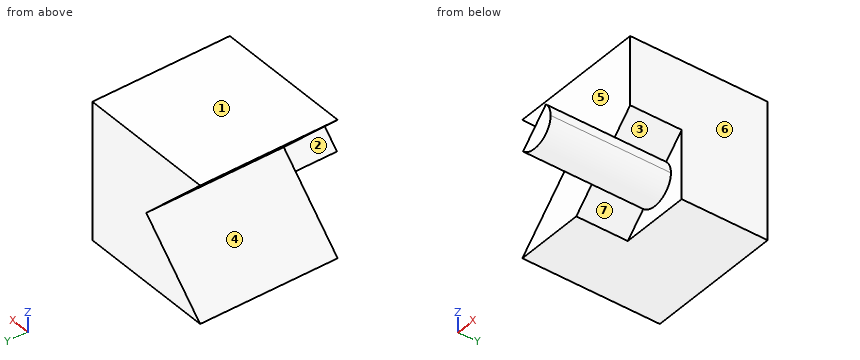
from build123d import *

# Parameters (mm, degrees)
F1_DEPTH = 40
F2_DEPTH = 25
F3_DEPTH = 60


with BuildPart() as f1:
    # F0 (on Front) → F1 (new body)
    with BuildSketch(Plane.XZ):
        with BuildLine():
            Line((20, 20), (0, 0))
            Line((0, 0), (20, 0))
            Line((20, 0), (25.7573593129, 5.7573593129))
            ThreePointArc((25.7573593129, 5.7573593129), (25.7573593129, 14.2426406871), (34.2426406871, 14.2426406871))
            Line((34.2426406871, 14.2426406871), (40, 20))
            Line((40, 20), (40, 40))
            Line((40, 40), (0, 40))
            Line((0, 40), (20, 20))
        make_face()
        with BuildLine():
            ThreePointArc((34.2426406871, 14.2426406871), (25.7573593129, 14.2426406871), (25.7573593129, 5.7573593129))
            Line((25.7573593129, 5.7573593129), (34.2426406871, 14.2426406871))
        make_face()
    extrude(amount=F1_DEPTH)

    # F0 (on Front) → F2 (join)
    with BuildSketch(Plane.XZ):
        with BuildLine():
            Line((25.7573593129, 5.7573593129), (20, 0))
            Line((20, 0), (40, 0))
            Line((40, 0), (40, 20))
            Line((40, 20), (34.2426406871, 14.2426406871))
            ThreePointArc((34.2426406871, 14.2426406871), (35.5432771951, 12.2961005942), (36, 10))
            ThreePointArc((36, 10), (32.2961005942, 4.4567228049), (25.7573593129, 5.7573593129))
        make_face()
    extrude(amount=F2_DEPTH)

    # F0 (on Front) → F3 (join)
    with BuildSketch(Plane.XZ):
        with BuildLine():
            Line((34.2426406871, 14.2426406871), (25.7573593129, 5.7573593129))
            ThreePointArc((25.7573593129, 5.7573593129), (32.2961005942, 4.4567228049), (36, 10))
            ThreePointArc((36, 10), (35.5432771951, 12.2961005942), (34.2426406871, 14.2426406871))
        make_face()
    extrude(amount=F3_DEPTH)


solid = f1.part
Verification items for the finished model (mm, model axes). Face numbers are marked on the shaded views. A direction names the side the tool comes from. Round coordinates to 2 decimals unless told otherwise and drop trailing zeros. Loops run counter-clockwise (first coordinate to the right, second up) from the corner with the lowest first, then second, coordinate; pieces in that order, holes last. Notation, with made-up numbers: (13.5, 86) - (72.5, 86) arc R20 cw to (72.5, 93) - close; hole circle Ø7 at (8.25, -24). An arc over 180 degrees is marked (long way). Use a Markdown table: item, result. Add a question column.
1. Section check C-C, the plane z = 16. Record the boundary of the cut face in (x, y).
2. Access from +Z, -Z, +X, -X, +Y, -Y to the whole of each face (thin tool, end or side, straight path). Record for the marked faces 1, 2, 3 and 4.
3. Gauge pin test, flat ends, axial feed: pin 1 (1 mm diameter, centred on y = -32.5, z = 7, fed in from -X); pin 2 (4 mm diameter, centred on y = -49.5, z = 11.5, fed in from -X); pin 3 (3 mm diameter, centred on y = -9, z = 28.5, fed in from -X). Record the tip position at first contact, or that the pin passes through.
4. Thickness scan on probe 1 along Y at (x, z) = (27.5, 9); probe 2 along Y at (x, z) = (35, 14.5); probe 3 along Z at (x, y) = (19, -23). Record the ranges inside material, lowest first. Write a range as [from, to].
5. Section check B-B, the plane y = -33. Record the boundary of the cut face in (x, z), plus the area to 3 significant figures.
6. Section check A-A, the plane x = 8. Record the boundary of the cut face in (y, z), plus the area to 3 significant figures.
7. Section check D-D, the plane x = 24.5. Record the boundary of the cut face in (y, z).
8. Release check for a two-part mould opening along X. For the marked faces 5, 6 and 7 record: released by +X, released by -X, zero draft, split by the parting line, or undercut.
Checks:
| question | item | result |
|---|---|---|
| 1 | outline | (16, -40) - (36, -40) - (36, -25) - (40, -25) - (40, 0) - (16, 0) - close |
| 2 | face 1 | +Z, +X, -X, +Y, -Y |
| 2 | face 2 | +Z, -X, -Y |
| 2 | face 3 | +X, -Y |
| 2 | face 4 | -X, +Y, -Y |
| 3 | pin 1 | stops at x = 6.5 |
| 3 | pin 2 | stops at x = 29.5 |
| 3 | pin 3 | stops at x = 10 |
| 4 | probe 1 | y = [-40, 0] |
| 4 | probe 2 | y = [-25, 0] |
| 4 | probe 3 | z = [0, 19], [21, 40] |
| 5 | outline | (0, 0) - (20, 0) - (25.76, 5.76) arc R6 ccw to (34.24, 14.24) - (40, 20) - (40, 40) - (0, 40) - (20, 20) - close |
| 5 | area | 1,060 mm^2 |
| 6 | outline | (-40, 0) - (0, 0) - (0, 8) - (-40, 8) - close; (-40, 32) - (0, 32) - (0, 40) - (-40, 40) - close |
| 6 | area | 640 mm^2 |
| 7 | outline | (-40, 4.5) - (-25, 4.5) - (-25, 0) - (0, 0) - (0, 40) - (-40, 40) - close |
| 8 | face 5 | zero draft |
| 8 | face 6 | released by +X |
| 8 | face 7 | undercut |
